Autodesk Inventor part; units mm, degrees
ref_plane "YZ Plane" through (0, 0, 0) normal (1, 0, 0) x (0, 1, 0)
ref_plane "XZ Plane" through (0, 0, 0) normal (0, 1, 0) x (-1, 0, 0)
ref_plane "XY Plane" through (0, 0, 0) normal (0, 0, 1) x (1, 0, 0)
sketch "Sketch1" plane through (0, 0, 0) normal (0, 0, 1) x (1, 0, 0)
  line L0 (-6.25, -7.25) -> (6.25, -7.25)
  line L1 (6.25, -7.25) -> (6.25, 7.25)
  line L2 (6.25, 7.25) -> (-6.25, 7.25)
  line L3 (-6.25, 7.25) -> (-6.25, -7.25)
  line L4 (-6.25, -7.25) -> (6.25, 7.25) construction
  line L5 (6.25, -7.25) -> (-6.25, 7.25) construction
  line L6 (-8.75, -9.75) -> (8.75, -9.75)
  line L7 (8.75, -9.75) -> (8.75, 9.75)
  line L8 (8.75, 9.75) -> (-8.75, 9.75)
  line L9 (-8.75, 9.75) -> (-8.75, -9.75)
  line L10 (-8.75, -9.75) -> (8.75, 9.75) construction
  line L11 (8.75, -9.75) -> (-8.75, 9.75) construction
  point P0 (0, 0)
  dimension "d0" = 12.5
  dimension "d1" = 14.5
  dimension "d2" = 17.5
  dimension "d3" = 19.5
extrude "Extrusion1" add sketch "Sketch1" along normal blind 10
sketch "Sketch2" plane through (0, 0, 0) normal (0, 0, -1) x (-1, 0, 0)
  line L0 (8.75, 9.75) -> (8.75, -9.75)
  line L1 (-8.75, 9.75) -> (8.75, 9.75)
  line L2 (8.75, 9.75) -> (8.75, 6.25)
  line L3 (8.75, 6.25) -> (-8.75, 6.25)
  line L4 (-8.75, 6.25) -> (-8.75, 9.75)
  line L5 (6.25, 7.25) -> (-6.25, 7.25)
  line L6 (-8.75, -9.75) -> (-8.75, 9.75)
  line L7 (-8.75, -9.75) -> (8.75, -9.75)
  line L8 (8.75, -9.75) -> (8.75, -6.25)
  line L9 (8.75, -6.25) -> (-8.75, -6.25)
  line L10 (-8.75, -6.25) -> (-8.75, -9.75)
  line L11 (-6.25, -7.25) -> (6.25, -7.25)
  point P0 (0, 0)
  point P1 (-8.75, -6.25)
  dimension "d6" = 1
  dimension "d7" = 1
extrude "Extrusion2" add sketch "Sketch2" along normal blind 2.5 contours L0 L3 L4 L1 | L0 L7 L6 L9
properties part number "Adafruit_1528_4663-ND_House_02"
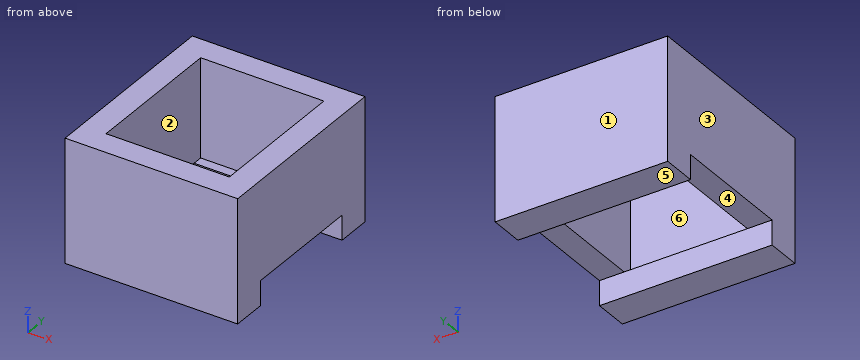
Input: part model. Units: mm. Frame: model coordinates. Face numbers are marked on the shaded views. A direction names the side the tool comes from. Give positions to 0.01 mm unless a question says otherwise; leave off trailing zeros. Write each loop counter-clockwise with the first axis right and the second up, starting at its lowest first coordinate (ties: lowest second). Pieces come first, ordered by that corner, then holes. Notation, with made-up numbers: (68.5, 21) - (95.5, 21) arc R32 ccw to (95.5, 49) - close; hole circle Ø3 at (15.5, 16). An arc over 180 degrees is marked (long way). Write item = value, one per line. Start each with the question number.
1. First-contact query: pin 1 Ø3 at (x, y) = (7, 1.5) entering from -Z; pin 2 Ø1 at (y, z) = (4, -1) entering from -X; pin 3 Ø0.8 at (x, y) = (1, 7) entering from +Z. Flat tips, straight axial feed; report the tip coordinate or a pass-through.
2. Section query D-D, the plane z = -1.5. Output: boundary loops of the cut face in (x, y).
3. Section query C-C, the plane z = 8. Output: boundary loops of the cut face in (x, y), then the cut area to 3 significant figures.
4. Section query A-A, the plane x = 0.75. Output: boundary loops of the cut face in (y, z), then the cut area to 3 significant figures.
5. Section query B-B, the plane y = 3.5. Output: boundary loops of the cut face in (x, z).
6. Access query for the marked faces 4, 5 and 6. Directions: +Z, -Z, +X, -X, +Y, -Y. A direction counts if a zero-diameter tool reaches every point of the face in a straight line with its end or side. Return the directions, or none.
7. Ray query, L1, parallel to Y at x = 3.5, z = 9; L2, parallel to X at y = 2.25, z = 5.75; L3, parallel to Y at x = 5.5, z = -1.5. Return the intervals inside material, ascending.
8. Mould query, pull axis X, two halves, no side actions, for the marked faces 1, 2 and 3. Classes: released by +X, released by -X, zero draft, split by the parting line, or undercut.
Check sheet entries:
q1.pin_1 = 0
q1.pin_2 = through
q1.pin_3 = 10
q2.outline = (-8.75, -9.75) - (8.75, -9.75) - (8.75, -6.25) - (-8.75, -6.25) - close; (-8.75, 6.25) - (8.75, 6.25) - (8.75, 9.75) - (-8.75, 9.75) - close
q3.outline = (-8.75, -9.75) - (8.75, -9.75) - (8.75, 9.75) - (-8.75, 9.75) - close; hole (-6.25, -7.25) - (6.25, -7.25) - (6.25, 7.25) - (-6.25, 7.25) - close
q3.area = 160 mm2
q4.outline = (-9.75, -2.5) - (-6.25, -2.5) - (-6.25, 0) - (-7.25, 0) - (-7.25, 10) - (-9.75, 10) - close; (6.25, -2.5) - (9.75, -2.5) - (9.75, 10) - (7.25, 10) - (7.25, 0) - (6.25, 0) - close
q4.area = 67.5 mm2
q5.outline = (-8.75, 0) - (-6.25, 0) - (-6.25, 10) - (-8.75, 10) - close; (6.25, 0) - (8.75, 0) - (8.75, 10) - (6.25, 10) - close
q6.face_4 = -Z, +X, -X
q6.face_5 = -Z, +X, -X, +Y, -Y
q6.face_6 = +Z
q7.L1 = -9.75 to -7.25, 7.25 to 9.75
q7.L2 = -8.75 to -6.25, 6.25 to 8.75
q7.L3 = -9.75 to -6.25, 6.25 to 9.75
q8.face_1 = zero draft
q8.face_2 = undercut
q8.face_3 = released by -X
